Check sheet for the modelled part. Datum: model origin and axes. Units: mm. Face numbers are marked on the shaded views. A direction names the side the tool comes from. Round coordinates to 2 decimals unless told otherwise and drop trailing zeros. Order: outer loops, then holes, each group sorted by start corner. A loop starts at its lowest first (then second) coordinate and runs counter-clockwise, first axis right, second up. Notation, with made-up numbers: (30, -24) -> (70, -24) arc R24 cw to (70, -3) -> close; hole circle Ø6 at (-17.75, -8). An arc over 180 degrees is marked (long way). Answer in a Markdown table with one row per item.
Autodesk Inventor part; units mm, degrees
ref_plane "YZ Plane" through (0, 0, 0) normal (1, 0, 0) x (0, 1, 0)
ref_plane "XZ Plane" through (0, 0, 0) normal (0, 1, 0) x (-1, 0, 0)
ref_plane "XY Plane" through (0, 0, 0) normal (0, 0, 1) x (1, 0, 0)
sketch "Sketch1" plane through (0, 0, 0) normal (0, 1, 0) x (-1, 0, 0)
  circle A0 centre (0, 0) radius 7.5
  line L0 (0, 3.75) -> (-24, 3.75)
  line L1 (-24, 3.75) -> (-24, -3.75)
  line L2 (-24, -3.75) -> (0, -3.75)
  line L3 (0, -3.75) -> (0, 3.75)
  circle A1 centre (-24, 0) radius 3.75
  line L4 (15, 14.5) -> (-34, 14.5)
  line L5 (-34, 14.5) -> (-34, -14.5)
  line L6 (-34, -14.5) -> (15, -14.5)
  line L7 (15, -14.5) -> (15, 14.5)
  point P0 (-6.4952, 3.75)
  point P1 (-6.4952, -3.75)
  dimension "d0" = 15
  dimension "d1" = 24
  dimension "d2" = 7.5
  dimension "d3" = 3.75
  dimension "d4" = 7
  dimension "d5" = 7
  dimension "d6" = 15
  dimension "d7" = 10
extrude "Extrusion1" add sketch "Sketch1" along normal blind 10
fillet "Fillet1" radius 4 2 edges at (6.4952, 5, 3.75) (6.4952, 5, -3.75)
sketch "Sketch2" plane through (0, 10, 0) normal (0, 1, 0) x (1, 0, 0)
  line L0 (-15, 14.5) -> (-15, -14.5)
  line L1 (34, -14.5) -> (34, 14.5)
  line L2 (-15, -14.5) -> (34, -14.5)
  line L3 (34, -14.5) -> (34, 14.5)
  line L4 (34, 14.5) -> (-15, 14.5)
  line L5 (-15, 14.5) -> (-15, -14.5)
  point P0 (0, 0)
extrude "Extrusion2" add sketch "Sketch2" along normal blind 2
sketch "Sketch3" plane through (0, 10, 0) normal (0, -1, 0) x (1, 0, 0)
  circle A0 centre (0, 0) radius 2
  arc A1 (24, -3.75) -> (24, 3.75) centre (24, 0) ccw
  circle A2 centre (24, 0) radius 1.5
  dimension "d13" = 4
  dimension "d14" = 3
extrude "Extrusion3" cut sketch "Sketch3" against normal blind 2
properties part number "servoTest"
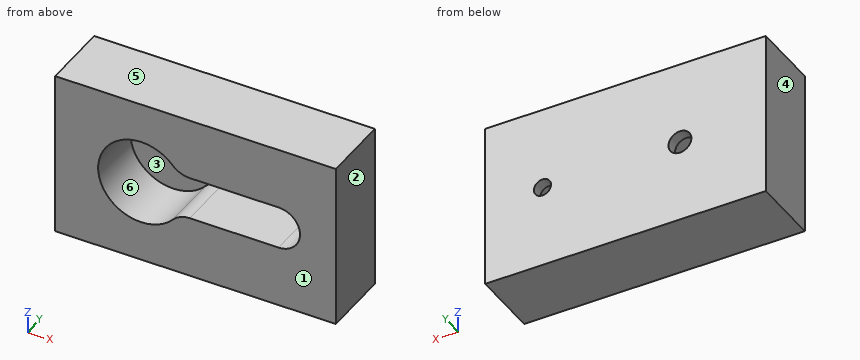
(1) Section check B-B on x = 0. Record the boundary of the cut face in (y, z), plus the area to 3 significant figures.
Solutions:
| item | result |
|---|---|
| outline | (0, -14.5) -> (12, -14.5) -> (12, -2) -> (10, -2) -> (10, -7.5) -> (0, -7.5) -> close; (0, 7.5) -> (10, 7.5) -> (10, 2) -> (12, 2) -> (12, 14.5) -> (0, 14.5) -> close |
| area | 190 mm^2 |
(2) Scan lines: probe 1 along Z at (x, y) = (16, 5.25); probe 2 along Z at (x, y) = (24, 10.6); probe 3 along X at (y, z) = (6, 0). Record each from-to range of solid material in increasing order. Write a range as from..to.
Solutions:
| item | result |
|---|---|
| probe 1 | -14.5..-3.75, 3.75..14.5 |
| probe 2 | -14.5..-1.5, 1.5..14.5 |
| probe 3 | -15..-7.5, 27.75..34 |
(3) Draft check along X on the marked faces 1, 2, 3 and 4. Enter one of: pulls with the +X half, pulls with the -X half, needs draft (parallel to the pull), parting line crosses it, or undercut.
Solutions:
| item | result |
|---|---|
| face 1 | needs draft |
| face 2 | pulls with the +X half |
| face 3 | undercut |
| face 4 | pulls with the -X half |
(4) Tool access check on the marked faces 5 and 6. Record the directions out of +Z, -Z, +X, -X, +Y, -Y that give a thin tool (end or side, any length) a straight path to the whole face; none if there is none.
Solutions:
| item | result |
|---|---|
| face 5 | +Z, +X, -X, +Y, -Y |
| face 6 | -Y |
(5) Section check D-D on x = 16. Record the boundary of the cut face in (y, z).
Solutions:
| item | result |
|---|---|
| outline | (0, -14.5) -> (12, -14.5) -> (12, 14.5) -> (0, 14.5) -> (0, 3.75) -> (10, 3.75) -> (10, -3.75) -> (0, -3.75) -> close |
(6) Section check A-A on z = 0. Record the boundary of the cut face in (x, y).
Solutions:
| item | result |
|---|---|
| outline | (-15, 0) -> (-7.5, 0) -> (-7.5, 10) -> (-2, 10) -> (-2, 12) -> (-15, 12) -> close; (2, 10) -> (22.5, 10) -> (22.5, 12) -> (2, 12) -> close; (25.5, 10) -> (27.75, 10) -> (27.75, 0) -> (34, 0) -> (34, 12) -> (25.5, 12) -> close |
(7) Section check C-C on y = 3. Record the boundary of the cut face in (x, z).
Solutions:
| item | result |
|---|---|
| outline | (-15, -14.5) -> (34, -14.5) -> (34, 14.5) -> (-15, 14.5) -> close; hole (5.54, -5.05) arc R4 cw to (8.5, -3.75) -> (24, -3.75) arc R3.75 ccw to (24, 3.75) -> (8.5, 3.75) arc R4 cw to (5.54, 5.05) arc R7.5 ccw (long way) to start |
